from build123d import *

# Parameters (mm, degrees)
F0_W      = 76.2
F0_H      = 76.2
F0_W_2    = 63.5
F0_H_2    = 63.5
F1_DEPTH  = 609.6
F2_W      = 177.8
F2_H      = 152.4
F3_DEPTH  = 12.7
F5_DEPTH  = 6.35
F6_W      = 6.35
F6_H      = 76.2
F7_DEPTH  = 44.45
F8_W      = 6.35
F8_H      = 76.2
F9_DEPTH  = 44.45
F10_R     = 4.7625
F11_DEPTH = 254
F13_W     = 25.4
F13_H     = 25.4
F14_DEPTH = 152.4
F15_W     = 50.8
F15_H     = 101.6
F16_DEPTH = 9.525
F17_W     = 50.8
F17_H     = 101.6
F18_DEPTH = 9.525
F19_R     = 4.7625
F20_DEPTH = 25.4
F21_R     = 4.7625
F22_DEPTH = 25.4


with BuildPart() as f1:
    # F0 (on Top) → F1 (new body)
    with BuildSketch(Plane.XY):
        Rectangle(F0_W, F0_H)
        Rectangle(F0_W_2, F0_H_2, mode=Mode.SUBTRACT)
    extrude(amount=F1_DEPTH)

    # F2 (on face) → F3 (join)
    with BuildSketch(Plane.XY.offset(609.6)):
        Rectangle(F2_W, F2_H)
    extrude(amount=F3_DEPTH)

    # F4 (on face) → F5 (join)
    with BuildSketch(Plane(origin=(0, 0, 609.6), x_dir=(1, 0, 0), z_dir=(0, 0, -1))):
        Polygon((95.25, 76.2), (88.9, 76.2), (44.45, 76.2), (44.45, 0), (95.25, 0), align=None)
        Polygon((-44.45, 76.2), (-88.9, 76.2), (-95.25, 76.2), (-95.25, 0), (-44.45, 0), align=None)
    extrude(amount=F5_DEPTH)

    # F6 (on face) → F7 (join)
    with BuildSketch(Plane.XY.offset(609.6)):
        with Locations((-92.075, -38.1)):
            Rectangle(F6_W, F6_H)
    extrude(amount=F7_DEPTH)

    # F8 (on face) → F9 (join)
    with BuildSketch(Plane.XY.offset(609.6)):
        with Locations((92.075, -38.1)):
            Rectangle(F8_W, F8_H)
    extrude(amount=F9_DEPTH)

    # F10 (on face) → F11 (cut)
    with BuildSketch(Plane.YZ.offset(95.25)):
        with Locations((-57.15, 635)):
            Circle(F10_R)
        with Locations((-19.05, 635)):
            Circle(F10_R)
    extrude(amount=-F11_DEPTH, mode=Mode.SUBTRACT)

    # F13 (on face) → F14 (join)
    with BuildSketch(Plane.XY.offset(622.3)):
        with Locations((-76.2, 63.5)):
            Rectangle(F13_W, F13_H)
        with Locations((76.2, 63.5)):
            Rectangle(F13_W, F13_H)
    extrude(amount=F14_DEPTH)

    # F15 (on face) → F16 (join)
    with BuildSketch(Plane.XY.offset(774.7)):
        with Locations((63.5, 101.6)):
            Rectangle(F15_W, F15_H)
    extrude(amount=F16_DEPTH)

    # F17 (on face) → F18 (join)
    with BuildSketch(Plane.XY.offset(774.7)):
        with Locations((-63.5, 101.6)):
            Rectangle(F17_W, F17_H)
    extrude(amount=F18_DEPTH)

    # F19 (on face) → F20 (cut)
    with BuildSketch(Plane.XY.offset(784.225)):
        with Locations((-47.625, 63.5)):
            Circle(F19_R)
        with Locations((-47.625, 139.7)):
            Circle(F19_R)
    extrude(amount=-F20_DEPTH, mode=Mode.SUBTRACT)

    # F21 (on face) → F22 (cut)
    with BuildSketch(Plane.XY.offset(784.225)):
        with Locations((47.625, 63.5)):
            Circle(F21_R)
        with Locations((47.625, 139.7)):
            Circle(F21_R)
    extrude(amount=-F22_DEPTH, mode=Mode.SUBTRACT)


solid = f1.part
Design review of the part built by this model. Coordinates are the model's own, in mm. A direction names the side the tool comes from. Round coordinates to 2 decimals unless told otherwise and drop trailing zeros. Write each loop counter-clockwise with the first axis right and the second up, starting at its lowest first coordinate (ties: lowest second). Pieces come first, ordered by that corner, then holes. Notation, with made-up numbers: M 79.5,78 L 115.5,78 A17 cw 115.5,88 Z; hole C 52,-2.5 d5. An arc over 180 degrees is marked long. One line per item, written item: value. Start each with the question number.
1. Take a section at C-C on x = 7.5. State the section outline as (y, z) points, then the cut area to 3 significant figures.
2. Draft analysis for pull direction X (two halves, no side actions). For faces 6 (the face through (88.9, 65, 697)), 7 (the face through (-64, 102, 784.225)), 8 (the face through (-88.9, 65, 697)), 9 (the face through (-1, 1, 622.3)), state which applies: pulls with the +X half, pulls with the -X half, needs draft (parallel to the pull), parting line crosses it, or undercut.
3. To check wall thickness, follow probe 1 along Y at (x, z) = (-91.25, 635); probe 2 along Z at (x, y) = (-90.5, -19.05); probe 3 along X at (y, z) = (-20, 368.5). State the ranges of each line that lie inside material, in increasing order. Write a range as from..to.
4. Take a section at A-A on z = 693.5. State the section outline as (x, y) points, then the cut area to 3 significant figures.
5. Take a section at B-B on z = 315. State the section outline as (x, y) points.
6. For faces 1 (the face through (-63.5, 63, 697)), 2 (the face through (0, 31.75, 301)), 3 (the face through (-70, -39, 603.25)), 4 (the face through (88.9, -39, 638)), 5 (the face through (63, 102, 774.7)), list the 3-axis set-ups (+Z, -Z, +X, -X, +Y, -Y) from which the entire face can be reached by the end or side of a thin tool; tool diameter is ignored.
7. Clearance check with flat-ended pins moving along their axes: P1, Ø3, axis at y = 7.5, z = 494.5, coming from the -X side; P2, Ø23, axis at x = 7.5, z = 185, coming from the +Y side; P3, Ø12, axis at x = 6, y = 4, coming from the -Z side. State where each tip first meets the part, or that it passes through.
Computed:
1. outline: M -76.2,609.6 L -38.1,609.6 L -38.1,0 L -31.75,0 L -31.75,609.6 L 31.75,609.6 L 31.75,0 L 38.1,0 L 38.1,609.6 L 76.2,609.6 L 76.2,622.3 L -76.2,622.3 Z
1. area: 9,680 mm²
2. face 6: pulls with the +X half
2. face 7: needs draft
2. face 8: pulls with the -X half
2. face 9: undercut
3. probe 1: y = -76.2..-61.91, -52.39..-23.81, -14.29..0
3. probe 2: z = 603.25..630.24, 639.76..654.05
3. probe 3: x = -38.1..-31.75, 31.75..38.1
4. outline: M -88.9,50.8 L -63.5,50.8 L -63.5,76.2 L -88.9,76.2 Z; M 63.5,50.8 L 88.9,50.8 L 88.9,76.2 L 63.5,76.2 Z
4. area: 1,290 mm²
5. outline: M -38.1,-38.1 L 38.1,-38.1 L 38.1,38.1 L -38.1,38.1 Z; hole M -31.75,-31.75 L 31.75,-31.75 L 31.75,31.75 L -31.75,31.75 Z
6. face 1: +Y, -Y
6. face 2: -Z
6. face 3: -Z, -X, +Y, -Y
6. face 4: +Z, -Y
6. face 5: +Y
7. P1: stops at x = -38.1
7. P2: stops at y = 38.1
7. P3: stops at z = 609.6
